Autodesk Inventor part; units mm, degrees
ref_plane "YZ Plane" through (0, 0, 0) normal (1, 0, 0) x (0, 1, 0)
ref_plane "XZ Plane" through (0, 0, 0) normal (0, 1, 0) x (-1, 0, 0)
ref_plane "XY Plane" through (0, 0, 0) normal (0, 0, 1) x (1, 0, 0)
sketch "Boceto1" plane through (0, 0, 0) normal (0, 1, 0) x (-1, 0, 0)
  point P0 (0, 0)
sketch "Boceto2" plane through (0, 0, 0) normal (0, 1, 0) x (-1, 0, 0)
  line L0 (-25, 38) -> (25, 38)
  line L1 (25, 38) -> (25, -38)
  line L2 (25, -38) -> (-25, -38)
  line L3 (-25, -38) -> (-25, 38)
  line L4 (-25, 38) -> (25, -38) construction
  line L5 (25, 38) -> (-25, -38) construction
  line L6 (28, -37) -> (28, 37)
  line L7 (24, 41) -> (-24, 41)
  line L8 (-28, 37) -> (-28, -37)
  line L9 (-24, -41) -> (24, -41)
  arc A0 (28, 37) -> (24, 41) centre (24, 37) ccw
  arc A1 (-24, 41) -> (-28, 37) centre (-24, 37) ccw
  arc A2 (-28, -37) -> (-24, -41) centre (-24, -37) ccw
  arc A3 (24, -41) -> (28, -37) centre (24, -37) ccw
  point P0 (0, 0)
  dimension "d0" = 50
  dimension "d1" = 76
  dimension "d2" = 3
  dimension "d3" = 4
extrude "Extrusión1" add sketch "Boceto2" along normal blind 14
sketch "Boceto3" plane through (0, 14, 0) normal (0, 1, 0) x (1, 0, 0)
  arc A0 (-28, -37) -> (-24, -41) centre (-24, -37) ccw
  line L0 (-24, -41) -> (24, -41)
  arc A1 (24, -41) -> (28, -37) centre (24, -37) ccw
  line L1 (28, -37) -> (28, 37)
  arc A2 (28, 37) -> (24, 41) centre (24, 37) ccw
  line L2 (24, 41) -> (-24, 41)
  arc A3 (-24, 41) -> (-28, 37) centre (-24, 37) ccw
  line L3 (-28, 37) -> (-28, -37)
  line L4 (25, -38) -> (-25, -38)
  line L5 (-25, -38) -> (-25, 38)
  line L6 (-25, 38) -> (25, 38)
  line L7 (25, 38) -> (25, -38)
  point P0 (0, 0)
extrude "Extrusión2" add sketch "Boceto3" along normal blind 1 contours L3 A3 L2 A2 L1 A1 L0 A0 | L4 L5 L6 L7
sketch "Boceto4" plane through (-25, 0, -38) normal (0, 0, 1) x (1, 0, 0)
  line L0 (0, 0) -> (50, 0)
  line L1 (50, 0) -> (50, 14)
  line L2 (0, 14) -> (50, 14)
  line L3 (0, 0) -> (0, 14)
  line L4 (0, 14) -> (10, 14)
  line L5 (10, 14) -> (14, 14)
  line L6 (14, 14) -> (14, 9)
  line L7 (14, 9) -> (10, 9)
  line L8 (10, 9) -> (10, 14)
  line L9 (14, 9) -> (21.5, 9)
  line L10 (21.5, 9) -> (21.5, 14)
  line L11 (21.5, 14) -> (14, 14)
  line L12 (14, 14) -> (14, 9)
  point P0 (25, 0)
  dimension "d8" = 10
  dimension "d9" = 4
  dimension "d10" = 5
  dimension "d11" = 7.5
  dimension "d12" = 5
extrude "Extrusión3" cut sketch "Boceto4" against normal through all contours L10 L9 L6 L2
sketch "Boceto5" plane through (-25, 0, -38) normal (0, 0, 1) x (1, 0, 0)
  line L0 (21.5, 14) -> (21.5, 9)
  line L1 (21.5, 9) -> (14, 9)
  line L2 (14, 9) -> (14, 14)
  line L3 (0, 14) -> (14, 14)
  line L4 (0, 0) -> (0, 14)
  line L5 (0, 0) -> (50, 0)
  line L6 (50, 0) -> (50, 14)
  line L7 (21.5, 14) -> (50, 14)
  line L8 (14, 9) -> (8, 9)
  line L9 (8, 9) -> (8, 14)
  line L10 (8, 14) -> (14, 14)
  line L11 (14, 14) -> (14, 9)
  line L12 (21.5, 14) -> (27.5, 14)
  line L13 (27.5, 14) -> (27.5, 9)
  line L14 (27.5, 9) -> (21.5, 9)
  line L15 (21.5, 9) -> (21.5, 14)
  point P0 (25, 0)
  dimension "d15" = 6
  dimension "d16" = 6
extrude "Extrusión4" add sketch "Boceto5" along normal blind 7 contours L7 L13 L14 L0 | L8 L9 L3 L2
sketch "Boceto6" plane through (0, 14, 0) normal (0, -1, 0) x (1, 0, 0)
  line L0 (-3.5, -41) -> (-3.5, -31)
  line L1 (-3.5, -31) -> (2.5, -31)
  line L2 (2.5, -31) -> (2.5, -38)
  line L3 (2.5, -38) -> (25, -38)
  line L4 (25, -38) -> (25, 38)
  line L5 (25, 38) -> (-25, 38)
  line L6 (-25, 38) -> (-25, -38)
  line L7 (-25, -38) -> (-17, -38)
  line L8 (-17, -38) -> (-17, -31)
  line L9 (-17, -31) -> (-11, -31)
  line L10 (-11, -31) -> (-11, -41)
  line L11 (-3.5, -41) -> (-11, -41)
  line L12 (-3.5, -31) -> (-11, -31)
  point P0 (0, 0)
extrude "Extrusión5" cut sketch "Boceto6" against normal blind 7 contours L11 L10 L12 L0
sketch "Boceto7" plane through (-3.5, 9, -38) normal (0, -1, 0) x (1, 0, 0)
  line L0 (-7.5, 0) -> (-13.5, 0)
  line L1 (-7.5, 0) -> (-7.5, 7)
  line L2 (-13.5, 7) -> (-7.5, 7)
  line L3 (-13.5, 0) -> (-13.5, 7)
  line L4 (6, 0) -> (0, 0)
  line L5 (6, 0) -> (6, 7)
  line L6 (0, 7) -> (6, 7)
  line L7 (0, 0) -> (0, 7)
  circle A0 centre (-11.25, 3) radius 0.75
  circle A1 centre (3.75, 3) radius 0.75
  point P0 (3.5, 38)
  dimension "d21" = 1.5
  dimension "d22" = 1.5
  dimension "d23" = 15
  dimension "d24" = 2.25
  dimension "d25" = 2.25
  dimension "d30" = 4
  dimension "d31" = 3
  dimension "d32" = 3
  dimension "d33" = 4
extrude "Extrusión6" cut sketch "Boceto7" against normal blind 3 contours A0 | A1
sketch "Boceto8" plane through (-25, 0, -31) normal (0, 0, 1) x (1, 0, 0)
  line L0 (14, 9) -> (14, 14)
  line L1 (8, 14) -> (14, 14)
  line L2 (8, 14) -> (8, 9)
  line L3 (8, 9) -> (14, 9)
  line L4 (27.5, 9) -> (27.5, 14)
  line L5 (21.5, 14) -> (27.5, 14)
  line L6 (21.5, 14) -> (21.5, 9)
  line L7 (21.5, 9) -> (27.5, 9)
  line L8 (14, 9) -> (8, 9)
  line L9 (14, 9) -> (21.5, 9)
  line L10 (21.5, 9) -> (21.5, 14)
  line L11 (21.5, 14) -> (14, 14)
  line L12 (14, 14) -> (14, 9)
  point P0 (25, 0)
extrude "Extrusión7" add sketch "Boceto8" along normal mid plane 1
properties part number "Pieza2_3DPrint"
Can you work these out from the model? Positions are in its coordinate system, mm. A direction names the side the tool comes from. Give positions to 0.01 mm unless a question says otherwise; leave off trailing zeros. Loops run counter-clockwise (first coordinate to the right, second up) from the corner with the lowest first, then second, coordinate; pieces in that order, holes last. Notation, with made-up numbers: M -4.5,48 L 40.5,48 A23 ccw 40.5,69 Z; hole C 30,-30 d2. An arc over 180 degrees is marked long. Use CSV: the item, a comma, the result in double quotes. Start each with the question number.
1. If I drill on L1, parallel to X at y = 10.8, z = -35; L2, parallel to Z at x = 12.5, y = 4; L3, parallel to Z at x = 0.25, y = 11.4, over which ranges is the centre line in solid material (lowest first)?
2. For P1, Ø3.5, axis at x = -8.5, z = -39.5, coming from the +Y side; P2, Ø6, axis at x = 6.5, z = -7.5, coming from the -Y side; P3, Ø1.4, axis at x = 0.25, z = -35, coming from the -Y side; P4, Ø2, axis at x = -8.5, z = -34.5, coming from the -Y side, each with a flat end and sliding along its axis, tell me the tip position at first contact or that it passes through.
3. Imagine slicing it at D-D, the plane y = 5.75. Write out the boundary of the cut face in (x, z), plus the area to 3 significant figures.
4. Imagine slicing it at B-B, the plane z = -5.5. Write out the boundary of the cut face in (x, y), plus the area to 3 significant figures.
5. Imagine slicing it at C-C, the plane x = -2. Write out the boundary of the cut face in (y, z), plus the area to 4 significant figures.
6. On a 3-axis mill with a long thin cutter (end or side, diameter ignored), from which of +Z, -Z, +X, -X, +Y, -Y can I reach the whole of each face in a straight line? I mean faces 1 (the face through (-3.5, 12, -36)), 2 (the face through (27, 0, -3)), 3 (the face through (-26.859, 7.395, -39.797)), 4 (the face through (-7, 12, -31.5)), 5 (the face through (-17, 11, -34)). Say none if no direction works.
7. If we mould it in two halves opening along Z, with no side actions, what happens to faces 6 (the face through (0, 14, 1)), 7 (the face through (-26.797, 7.395, 39.859)), 8 (the face through (-7, 12, -30.5)), 9 (the face through (-7, 9, -39))? For each: released by +Z, released by -Z, zero draft, split by the parting line, or undercut.
8. Imagine slicing it at A-A, the plane y = 13. Write out the boundary of the cut face in (x, z).
Response values:
1,L1,"-28 to -25, -17 to -15.5, -14 to -11, -3.5 to -0.5, 1 to 2.5, 25 to 28"
1,L2,"-41 to -38, 38 to 41"
1,L3,"-41 to -35.75, -34.25 to -30.5, 38 to 41"
2,P1,"y = 9"
2,P2,"y = 14"
2,P3,"y = 12"
2,P4,"through"
3,outline,"M -28,-37 A4 ccw -24,-41 L 24,-41 A4 ccw 28,-37 L 28,37 A4 ccw 24,41 L -24,41 A4 ccw -28,37 Z; hole M -25,-38 L 25,-38 L 25,38 L -25,38 Z"
3,area,"778 mm^2"
4,outline,"M -28,0 L -25,0 L -25,14 L 25,14 L 25,0 L 28,0 L 28,15 L -28,15 Z"
4,area,"140 mm^2"
5,outline,"M 0,-41 L 15,-41 L 15,41 L 0,41 L 0,38 L 14,38 L 14,-30.5 L 9,-30.5 L 9,-38 L 0,-38 Z"
5,area,"203.5 mm^2"
6,face 1,"-Z, +Y"
6,face 2,"+Z, -Z, +X, -X, -Y"
6,face 3,"-Z, -X, +Y, -Y"
6,face 4,"-Z, +Y, -Y"
6,face 5,"-Y"
7,face 6,"undercut"
7,face 7,"released by +Z"
7,face 8,"undercut"
7,face 9,"zero draft"
8,outline,"M -28,-37 A4 ccw -24,-41 L -11,-41 L -11,-31.5 L -3.5,-31.5 L -3.5,-41 L 24,-41 A4 ccw 28,-37 L 28,37 A4 ccw 24,41 L -24,41 A4 ccw -28,37 Z; hole M -25,-38 L -17,-38 L -17,-30.5 L 2.5,-30.5 L 2.5,-38 L 25,-38 L 25,38 L -25,38 Z"
